Design review of the part built by this model. Coordinates are the model's own, in mm. Round coordinates to 2 decimals unless told otherwise and drop trailing zeros. Order: outer loops, then holes, each group sorted by start corner. A loop starts at its lowest first (then second) coordinate and runs counter-clockwise, first axis right, second up. Notation, with made-up numbers: M -6,65 L 38,65 A18 cw 38,94 Z; hole C -36.5,83.25 d5. An arc over 180 degrees is marked long. Use a Markdown table: item, result. Add a question column.
(1) Take a section at A-A (x = 0). Write out the cut boundary in (y, z), then the cut area to 3 significant figures.
(2) Take a section at D-D (z = 4). Write out the cut boundary in (x, y), then the cut area to 3 significant figures.
(3) The part is to be moulded in two halves that separate along X. For faces 1 (the face through (0, 0, 6.05)), 2 (the face through (0, 0, 6.8)), 3 (the face through (-2.9, -13.05, 4.94)), say which applies: released by +X, released by -X, zero draft, split by the parting line, or undercut.
(4) Take a section at C-C (z = 1). Write out the cut boundary in (x, y).
(5) To check wall thickness, follow probe 1 along Z at (x, y) = (-3.5, -1.25); probe 2 along Y at (x, z) = (-0.25, 5.5); probe 3 along X at (y, z) = (9, 3.75). State the ranges of each line that lie inside material, in increasing order. Write a range as from..to.
(6) For pin 1 (2 mm diameter, centred on y = 11, z = 4, fed in from -X); pin 2 (1 mm diameter, centred on x = 7.5, z = 3.5, fed in from -Y); pin 3 (11.5 mm diameter, centred on x = -4, y = 0, fed in from -Z), all flat-tipped, find the tip position at first contact; note any pin that passes through.
```python
from build123d import *

# Parameters (mm, degrees)
F2_R = 2
F3_T = -0.75


with BuildPart() as f1:
    # F0 (on Front) → F1 (revolve)
    with BuildSketch(Plane.XZ):
        Polygon((0, 6.8), (0, 0), (14.35, 0), (13, 6.8), align=None)
    revolve(axis=Axis((0, 0, 3.4), (0, 0, 1)))

    # F2
    f2_edges = [f1.edges().sort_by_distance(p)[0] for p in [
        (-13, 0, 6.8),
    ]]
    fillet(f2_edges, radius=F2_R)

    # F3
    f3_openings = [f1.faces().sort_by_distance(p)[0] for p in [
        (0, 0, 0),
    ]]
    offset(amount=F3_T, openings=f3_openings)


solid = f1.part
```
Verdict:
| question | item | result |
|---|---|---|
| 1 | outline | M -14.35,0 L -13.59,0 L -12.58,5.04 A1.25 cw -11.36,6.05 L 11.36,6.05 A1.25 cw 12.58,5.04 L 13.59,0 L 14.35,0 L 13.32,5.19 A2 ccw 11.36,6.8 L -11.36,6.8 A2 ccw -13.32,5.19 Z |
| 1 | area | 28.2 mm^2 |
| 2 | outline | C 0,0 d27.11; hole C 0,0 d25.58 |
| 2 | area | 63.3 mm^2 |
| 3 | face 1 | undercut |
| 3 | face 2 | zero draft |
| 3 | face 3 | split by the parting line |
| 4 | outline | C 0,0 d28.3; hole C 0,0 d26.77 |
| 5 | probe 1 | z = 6.05..6.8 |
| 5 | probe 2 | y = -13.23..-12.39, 12.39..13.23 |
| 5 | probe 3 | x = -10.2..-9.16, 9.16..10.2 |
| 6 | pin 1 | stops at x = -9.19 |
| 6 | pin 2 | stops at y = -11.75 |
| 6 | pin 3 | stops at z = 6.05 |
